```python
from build123d import *

# Parameters (mm, degrees)
F0_W     = 50
F0_H     = 50
F1_DEPTH = 25.4
F3_D     = 20
F4_R     = 5
F6_D     = 5


with BuildPart() as f1:
    # F0 (on Front) → F1 (new body)
    with BuildSketch(Plane.XZ):
        with Locations((25, 25)):
            Rectangle(F0_W, F0_H)
    extrude(amount=F1_DEPTH)

    # F3 (through all)
    with Locations(Plane.XZ.offset(25.4)):
        with Locations((24.9791759998, 25.4528727382)):
            Hole(F3_D / 2)

    # F4
    f4_edges = [f1.edges().sort_by_distance(p)[0] for p in [
        (50, -12.7, 50),
        (50, -12.7, 0),
        (0, -12.7, 50),
        (0, -12.7, 0),
        (14.979176, 0, 25.452873),
        (14.979176, -25.4, 25.452873),
    ]]
    fillet(f4_edges, radius=F4_R)

    # F6 (through all)
    with Locations(Plane.XZ.offset(25.4)):
        with Locations((40.0353602501, 45.0723162054)):
            Hole(F6_D / 2)


solid = f1.part
```
The model under review builds one solid part; all positions refer to its coordinate system, in mm. Coordinates: 2 decimals unless noted, no trailing zeros. Write each loop counter-clockwise with the first axis right and the second up, starting at its lowest first coordinate (ties: lowest second). Pieces come first, ordered by that corner, then holes. Notation, with made-up numbers: (-2.75, 15.25) - (17.25, 15.25) arc R24 cw to (17.25, 34.25) - close; hole circle Ø5 at (-17.5, 6). An arc over 180 degrees is marked (long way). Answer in a Markdown table with one row per item. Add a question column.
Q1. Clearance check with a flat-ended pin moving along its axis: pin 1 (3 mm diameter, centred on x = 22.5, z = 36.5, fed in from -Y). State where the tip first meets the part, or that it passes through.
Q2. To check wall thickness, follow line 1 along Y through (x, z) = (35, 36.5); line 2 along Z through (x, y) = (34, -12); line 3 along X through (y, z) = (-12.25, 28). State the ranges of each line that lie inside material, in increasing order. Write a range as from..to.
Q3. Consider section A-A on y = -2.5. Give the boundary of the cut face in (x, z), then the cut area to 3 significant figures.
Q4. Consider section B-B on y = -22.75. Give the boundary of the cut face in (x, z), then the cut area to 3 significant figures.
Q5. Draft analysis for pull direction Z (two halves, no side actions). For faces 1 (the face through (38.69, -12.52, 47.18)), 2 (the face through (48, -13, 1)), 3 (the face through (48, -13, 49)), 4 (the face through (19.603, -12.592, 33.885)), state which applies: +Z half, -Z half, draft (parallel to the pull), parting line (faces both ways), or undercut.
Answers below:
| question | item | result |
|---|---|---|
| 1 | pin 1 | y = -24.9 |
| 2 | line 1 | -25.4..0 |
| 2 | line 2 | 0..21.14, 29.77..50 |
| 2 | line 3 | 0..15.31, 34.65..50 |
| 3 | outline | (0, 5) arc R5 ccw to (5, 0) - (45, 0) arc R5 ccw to (50, 5) - (50, 45) arc R5 ccw to (45, 50) - (5, 50) arc R5 ccw to (0, 45) - close; hole circle Ø21.34 at (24.98, 25.45); hole circle Ø5 at (40.04, 45.07) |
| 3 | area | 2,100 mm² |
| 4 | outline | (0, 5) arc R5 ccw to (5, 0) - (45, 0) arc R5 ccw to (50, 5) - (50, 45) arc R5 ccw to (45, 50) - (5, 50) arc R5 ccw to (0, 45) - close; hole circle Ø21.17 at (24.98, 25.45); hole circle Ø5 at (40.04, 45.07) |
| 4 | area | 2,110 mm² |
| 5 | face 1 | undercut |
| 5 | face 2 | -Z half |
| 5 | face 3 | +Z half |
| 5 | face 4 | undercut |
